For this review, take the finished solid that the model builds, in its own axes (mm). Face numbers are marked on the shaded views. A direction names the side the tool comes from. Round coordinates to 2 decimals unless told otherwise and drop trailing zeros. Order: outer loops, then holes, each group sorted by start corner. A loop starts at its lowest first (then second) coordinate and runs counter-clockwise, first axis right, second up. Notation, with made-up numbers: (39.5, 52) -> (60.5, 52) arc R23 ccw to (60.5, 67) -> close; hole circle Ø3 at (77, 64). An arc over 180 degrees is marked (long way). Answer in a Markdown table with one row per item.
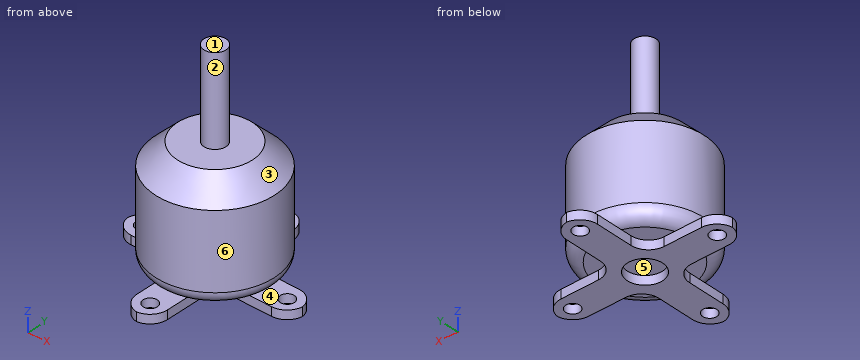
```python
from build123d import *

# Parameters (mm, degrees)
SKETCH1_R           = 13.5
BOSS_EXTRUDE1_DEPTH = 25
SKETCH2_R           = 2.5
BOSS_EXTRUDE2_DEPTH = 20
FILLET1_R           = 3
CHAMFER1_SIZE       = 5
SKETCH3_R           = 1.6
BOSS_EXTRUDE3_DEPTH = 2
SKETCH4_R           = 4
CUT_EXTRUDE1_DEPTH  = 2


with BuildPart() as part:
    # Sketch1 → Boss-Extrude1 (new body)
    with BuildSketch(Plane.XY):
        Circle(SKETCH1_R)
    extrude(amount=BOSS_EXTRUDE1_DEPTH)

    # Sketch2 → Boss-Extrude2 (add)
    with BuildSketch(Plane.XY.offset(25)):
        Circle(SKETCH2_R)
    extrude(amount=BOSS_EXTRUDE2_DEPTH)

    # Fillet1
    fillet1_edges = [part.edges().sort_by_distance(p)[0] for p in [
        (-13.5, 0, 0),
    ]]
    fillet(fillet1_edges, radius=FILLET1_R)

    # Chamfer1
    chamfer1_edges = [part.edges().sort_by_distance(p)[0] for p in [
        (-13.5, 0, 25),
    ]]
    chamfer(chamfer1_edges, length=CHAMFER1_SIZE)

    # Sketch3 → Boss-Extrude3 (add)
    with BuildSketch(Plane(origin=(0, 0, 0), x_dir=(-1, 0, 0), z_dir=(0, 0, -1))):
        with BuildLine():
            Line((-3.5, -7.5), (-3.5, -16))
            ThreePointArc((-3.5, -16), (-2.5, -18.645751311), (0, -19.968626967))
            ThreePointArc((0, -19.968626967), (2.5, -18.645751311), (3.5, -16))
            Line((3.5, -16), (3.5, -7.5))
            ThreePointArc((3.5, -7.5), (4.671572875, -4.671572875), (7.5, -3.5))
            Line((7.5, -3.5), (16, -3.5))
            ThreePointArc((16, -3.5), (18.645751311, -2.5), (19.968626967, 0))
            ThreePointArc((19.968626967, 0), (18.645751311, 2.5), (16, 3.5))
            Line((16, 3.5), (7.5, 3.5))
            ThreePointArc((7.5, 3.5), (4.671572875, 4.671572875), (3.5, 7.5))
            Line((3.5, 7.5), (3.5, 16))
            ThreePointArc((3.5, 16), (2.5, 18.645751311), (0, 19.968626967))
            ThreePointArc((0, 19.968626967), (-2.5, 18.645751311), (-3.5, 16))
            Line((-3.5, 16), (-3.5, 7.5))
            ThreePointArc((-3.5, 7.5), (-4.671572875, 4.671572875), (-7.5, 3.5))
            Line((-7.5, 3.5), (-16, 3.5))
            ThreePointArc((-16, 3.5), (-18.645751311, 2.5), (-19.968626967, 0))
            ThreePointArc((-19.968626967, 0), (-18.645751311, -2.5), (-16, -3.5))
            Line((-16, -3.5), (-7.5, -3.5))
            ThreePointArc((-7.5, -3.5), (-4.671572875, -4.671572875), (-3.5, -7.5))
        make_face()
        with Locations((-16.5, 0)):
            Circle(SKETCH3_R, mode=Mode.SUBTRACT)
        with Locations((0, 16.5)):
            Circle(SKETCH3_R, mode=Mode.SUBTRACT)
        with Locations((16.5, 0)):
            Circle(SKETCH3_R, mode=Mode.SUBTRACT)
        with Locations((0, -16.5)):
            Circle(SKETCH3_R, mode=Mode.SUBTRACT)
    extrude(amount=BOSS_EXTRUDE3_DEPTH)

    # Sketch4 → Cut-Extrude1 (cut)
    with BuildSketch(Plane(origin=(0, 0, -2), x_dir=(-1, 0, 0), z_dir=(0, 0, -1))):
        Circle(SKETCH4_R)
    extrude(amount=-CUT_EXTRUDE1_DEPTH, mode=Mode.SUBTRACT)


solid = part.part
```
Q1. Take a section at C-C, the plane z = 42.5. Write out the cut boundary in (x, y), then the cut area to 3 significant figures.
Answer key:
| item | result |
|---|---|
| outline | circle Ø5 at (0, 0) |
| area | 19.6 mm^2 |
Q2. Tool access review of the marked faces 1 and 2: name each direction out of +Z, -Z, +X, -X, +Y, -Y from which nothing blocks a thin tool from reaching the whole face with its end or side.
Answer key:
| item | result |
|---|---|
| face 1 | +Z, +X, -X, +Y, -Y |
| face 2 | +Z |
Q3. To check wall thickness, follow probe 1 along Y at (x, z) = (16.5, -1.25); probe 2 along Z at (x, y) = (-13.5, 2.5); probe 3 along Y at (x, z) = (0, 15). State the ranges of each line that lie inside material, in increasing order.
Answer key:
| item | result |
|---|---|
| probe 1 | y = -3.47 to -1.6, 1.6 to 3.47 |
| probe 2 | z = -2 to 0 |
| probe 3 | y = -13.5 to 13.5 |
Q4. Take a section at B-B, the plane x = 1. Give the number of separate pieces and of enclosed holes in the cut face, then the cut area to 3 significant figures.
Answer key:
| item | result |
|---|---|
| separate pieces | 3 |
| enclosed holes | 0 |
| area | 789 mm^2 |
Q5. Clearance check with flat-ended pins moving along their axes: pin 1 Ø1.6 at (y, z) = (11, -1) entering from +X; pin 2 Ø1.9 at (x, y) = (0, -16.5) entering from +Z; pin 3 Ø0.6 at (y, z) = (-10.5, -1) entering from -X; pin 4 Ø2 at (x, y) = (-1, 16.5) entering from +Z. State where each tip first meets the part, or that it passes through.
Answer key:
| item | result |
|---|---|
| pin 1 | stops at x = 3.5 |
| pin 2 | passes through |
| pin 3 | stops at x = -3.5 |
| pin 4 | stops at z = 0 |
Q6. The part is to be moulded in two halves that separate along Z. For the marked faces 3, 4, 5 and 6, say which applies: +Z half, -Z half, draft (parallel to the pull), parting line (faces both ways), or undercut.
Answer key:
| item | result |
|---|---|
| face 3 | +Z half |
| face 4 | undercut |
| face 5 | -Z half |
| face 6 | draft |
Q7. Take a section at A-A, the plane z = 5. Write out the cut boundary in (x, y), then the cut area to 3 significant figures.
Answer key:
| item | result |
|---|---|
| outline | circle Ø27 at (0, 0) |
| area | 573 mm^2 |
